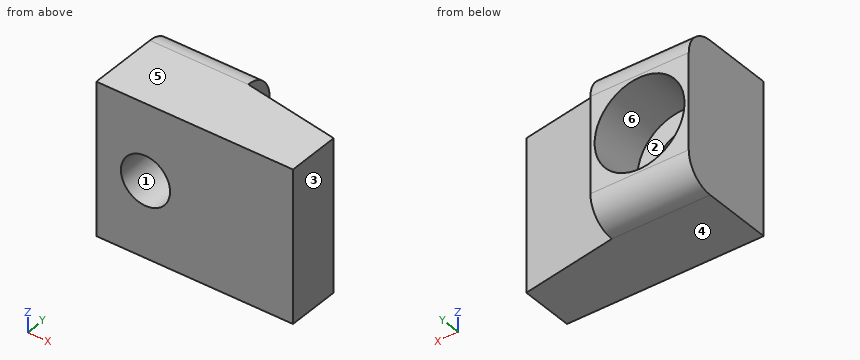
```python
from build123d import *

# Parameters (mm, degrees)
F1_DEPTH = 10.8
F2_R     = 1.75
F3_DEPTH = 7.001
F4_R     = 3.2
F5_DEPTH = 4
F6_R     = 2


with BuildPart() as f1:
    # F0 (on Top) → F1 (new body)
    with BuildSketch(Plane.XY):
        Polygon((-7, 7), (-7, 0), (7, 0), (7, 3.8), (0, 5), (0, 7), align=None)
    extrude(amount=F1_DEPTH)

    # F2 (on face) → F3 (cut, through all)
    with BuildSketch(Plane(origin=(0, 7, 0), x_dir=(-1, 0, 0), z_dir=(0, 1, 0))):
        with Locations((3.5, 5.4)):
            Circle(F2_R)
    extrude(amount=-F3_DEPTH, mode=Mode.SUBTRACT)

    # F4 (on face) → F5 (cut)
    with BuildSketch(Plane(origin=(0, 7, 0), x_dir=(-1, 0, 0), z_dir=(0, 1, 0))):
        with Locations((3.5, 5.4)):
            Circle(F4_R)
    extrude(amount=-F5_DEPTH, mode=Mode.SUBTRACT)

    # F6
    f6_edges = [f1.edges().sort_by_distance(p)[0] for p in [
        (-3.5, 7, 10.8),
        (-3.5, 7, 0),
    ]]
    fillet(f6_edges, radius=F6_R)


solid = f1.part
```
Geometry: final body of the model. Coordinates: model frame, mm. Face numbers are marked on the shaded views. A direction names the side the tool comes from. Round coordinates to 2 decimals unless told otherwise and drop trailing zeros. Loops run counter-clockwise (first coordinate to the right, second up) from the corner with the lowest first, then second, coordinate; pieces in that order, holes last.
Item 1: Section D-D, the plane x = -6. Output: boundary loops of the cut face in (y, z).
Checked values:
outline: (0, 0) - (5, 0) arc R2 ccw to (7, 2) - (7, 3.4) - (3, 3.4) - (3, 7.4) - (7, 7.4) - (7, 8.8) arc R2 ccw to (5, 10.8) - (0, 10.8) - close
Item 2: Mould query, pull axis Z, two halves, no side actions, for the marked faces 1, 2, 3 and 4. Classes: released by +Z, released by -Z, zero draft, split by the parting line, or undercut.
Checked values:
face 1: undercut
face 2: undercut
face 3: zero draft
face 4: released by -Z
Item 3: Line query: L1, parallel to Z at x = -3.5, y = 4.1; L2, parallel to Z at x = -3.5, y = 2.25; L3, parallel to X at y = 3.5, z = 4.75. Output: solid intervals per line, ascending.
Checked values:
L1: z = 0 to 2.2, 8.6 to 10.8
L2: z = 0 to 3.65, 7.15 to 10.8
L3: x = -7 to -6.63, -0.37 to 7
Item 4: Section A-A, the plane x = -3.5. Output: boundary loops of the cut face in (y, z), plus the area to 3 significant figures.
Checked values:
outline: (0, 0) - (5, 0) arc R2 ccw to (7, 2) - (7, 2.2) - (3, 2.2) - (3, 3.65) - (0, 3.65) - close; (0, 7.15) - (3, 7.15) - (3, 8.6) - (7, 8.6) - (7, 8.8) arc R2 ccw to (5, 10.8) - (0, 10.8) - close
area: 37.8 mm2
Item 5: Reachability of the marked faces 5 and 6 from +Z, -Z, +X, -X, +Y, -Y: full face, straight path, thin tool, end or side. Return the list, or none.
Checked values:
face 5: +Z, +X, -X, +Y, -Y
face 6: +Y
Item 6: Contact query for flat-ended pins moving along their axis: P1, Ø0.6, axis at y = 6, z = 3.5, coming from the +X side; P2, Ø1.9, axis at x = -4, z = 7, coming from the +Y side; P3, Ø4, axis at x = 2.5, z = 9.5, coming from the +Y side. Output: stop coordinate, or through.
Checked values:
P1: stops at x = 0
P2: stops at y = 3
P3: stops at y = 4.91
Item 7: Section C-C, the plane y = 2. Output: boundary loops of the cut face in (x, z), plus the area to 3 significant figures.
Checked values:
outline: (-7, 0) - (7, 0) - (7, 10.8) - (-7, 10.8) - close; hole circle Ø3.5 at (-3.5, 5.4)
area: 142 mm2
Item 8: Section B-B, the plane z = 5.4. Output: boundary loops of the cut face in (x, y), plus the area to 3 significant figures.
Checked values:
outline: (-7, 0) - (-5.25, 0) - (-5.25, 3) - (-6.7, 3) - (-6.7, 7) - (-7, 7) - close; (-1.75, 0) - (7, 0) - (7, 3.8) - (0, 5) - (0, 7) - (-0.3, 7) - (-0.3, 3) - (-1.75, 3) - close
area: 43.7 mm2
